Solid Edge part; units mm, degrees
sketch "Sketch1" plane through (0, 0, 0) normal (0, -1, 0) x (1, 0, 0)
  line L0 (0, 5) -> (3.75, 5)
  line L1 (3.75, 5) -> (4.25, 4.5)
  line L2 (4.25, 4.5) -> (4.25, 0)
  line L3 (4.25, 0) -> (2.5, 0)
  line L4 (2.5, 0) -> (2.5, -19.2)
  line L5 (2.5, -19.2) -> (1.7, -20)
  line L6 (1.7, -20) -> (0, -20)
  line L7 (0, -20) -> (0, 5)
  dimension "D1" = 2.5
  dimension "D2" = 3.75
revolve "RevolvedProtrusion1" add sketch "Sketch1" angle 360 about axis through (0, 0, 54) along (0, 0, -1)
sketch "Sketch2" plane through (0, 0, 5) normal (0, 0, 1) x (0, 1, 0)
  line L0 (-2.3094, 0) -> (-1.1547, 2)
  line L1 (-1.1547, 2) -> (1.1547, 2)
  line L2 (1.1547, 2) -> (2.3094, 0)
  line L3 (2.3094, 0) -> (1.1547, -2)
  line L4 (1.1547, -2) -> (-1.1547, -2)
  line L5 (-1.1547, -2) -> (-2.3094, 0)
extrude "Cutout1" cut sketch "Sketch2" against normal blind 2.5
cosmetic_thread "Thread1"
properties material "Steel"
Could you check a few things on this model? Use its own coordinates, in mm. A direction names the side the tool comes from. Round coordinates to 2 decimals unless told otherwise and drop trailing zeros. Order: outer loops, then holes, each group sorted by start corner. A loop starts at its lowest first (then second) coordinate and runs counter-clockwise, first axis right, second up.
Q1. I'm going to push flat-ended pins straight in: P1, Ø1.2, axis at y = 0.5, z = 4, coming from the +X side; P2, Ø5, axis at x = -2.5, z = -11, coming from the -Y side; P3, Ø2, axis at x = -2, y = -3, coming from the -Z side; P4, Ø1, axis at y = -1, z = 0, coming from the -X side. Where does each tip first touch, or does it pass through?
Geometry says:
P1: stops at x = 4.25
P2: stops at y = -2.5
P3: stops at z = 0
P4: stops at x = -4.22
Q2. Please list where these lines run through material, in increasing order: probe 1 along Z at (x, y) = (1.5, -0.25); probe 2 along X at (y, z) = (1.5, -1.25); probe 3 along Z at (x, y) = (-2, 1.75).
Geometry says:
probe 1: z = -20 to 2.5
probe 2: x = -2 to 2
probe 3: z = 0 to 5
Q3. Imagine slicing it at A-A, the plane y = 0. List the corners of the cut face in (x, z) for me.
Geometry says:
outline: (-4.25, 0) - (-2.5, 0) - (-2.5, -19.2) - (-1.7, -20) - (1.7, -20) - (2.5, -19.2) - (2.5, 0) - (4.25, 0) - (4.25, 4.5) - (3.75, 5) - (2, 5) - (2, 2.5) - (-2, 2.5) - (-2, 5) - (-3.75, 5) - (-4.25, 4.5) - close
Q4. Imagine slicing it at C-C, the plane z = -3.5. List the corners of the cut face in (x, y) for me, then the cut area to 3 significant figures.
Geometry says:
outline: circle Ø5 at (0, 0)
area: 19.6 mm2
Q5. Imagine slicing it at B-B, the plane z = 1.5. List the corners of the cut face in (x, y) for me.
Geometry says:
outline: circle Ø8.5 at (0, 0)
Q6. Thinking about a two-plate mould opening in X: for faces 4 (the face through (2.285, -3.584, 2.218)), 5 (the face through (0, 0, 2.5)), 6 (the face through (2, 2, 5)), which applies, released by +X, released by -X, zero draft, split by the parting line, or undercut?
Geometry says:
face 4: split by the parting line
face 5: undercut
face 6: zero draft
Q7. Which directions (+Z, -Z, +X, -X, +Y, -Y) give clear straight access to the entire face, cutting with the end or side of a thin tool? Please do faces 1 (the face through (-0.54, 2.44, -9.73)), 2 (the face through (0, 0, -20)), 3 (the face through (-2, 0, 4)).
Geometry says:
face 1: -Z
face 2: -Z, +X, -X, +Y, -Y
face 3: +Z
